from build123d import *

# Parameters (mm, degrees)
EXTRUDE1_DEPTH     = 50.8
SKETCH2_R          = 3.5687
CUT_EXTRUDE1_DEPTH = 7.3500001
SKETCH3_R          = 4.1656
CUT_EXTRUDE2_DEPTH = 128.0000001


with BuildPart() as part:
    # Sketch1 → Extrude1 (new body)
    with BuildSketch(Plane.XY):
        with BuildLine():
            Line((24.787766027, 20.626332144), (6.630852488, 23.827885887))
            Line((6.630852488, 23.827885887), (-1.306647512, 25.227481296))
            Line((-1.306647512, 25.227481296), (-11.14056344, 26.961466))
            add(Edge.make_bspline(
                [(-16.387897512, 33.214995232), (-16.387897512, 27.886712574), (-11.14056344, 26.961466)],
                knots=[1.570796327, 1.570796327, 1.570796327, 2.967059728, 2.967059728, 2.967059728], degree=2, weights=[1, 0.766044443, 1]))
            Line((-16.387897512, 33.214995232), (-16.387897512, 79.980278282))
            Line((-16.387897512, 79.980278282), (-16.387897512, 87.117678282))
            Line((-16.387897512, 87.117678282), (-16.387897512, 118.080278282))
            Line((-16.387897512, 118.080278282), (-16.387897512, 125.217678282))
            Line((-16.387897512, 125.217678282), (-16.387897512, 134.348978282))
            add(Edge.make_bspline(
                [(-16.387897512, 134.348978282), (-16.387897512, 140.698978282), (-22.737897512, 140.698978282)],
                knots=[3.141592654, 3.141592654, 3.141592654, 4.71238898, 4.71238898, 4.71238898], degree=2, weights=[1, 0.707106781, 1]))
            Line((-22.737897512, 140.698978282), (-22.737897512, 125.217678282))
            Line((-22.737897512, 125.217678282), (-22.737897512, 118.080278282))
            Line((-22.737897512, 118.080278282), (-22.737897512, 87.117678282))
            Line((-22.737897512, 87.117678282), (-22.737897512, 79.980278282))
            Line((-22.737897512, 79.980278282), (-22.737897512, 13.698978282))
            Line((-22.737897512, 13.698978282), (-1.306647512, 13.698978282))
            Line((-1.306647512, 13.698978282), (6.630852488, 13.698978282))
            Line((6.630852488, 13.698978282), (28.062102488, 13.698978282))
            Line((28.062102488, 13.698978282), (28.062102488, 16.724129903))
            add(Edge.make_bspline(
                [(28.062102488, 16.724129903), (28.062102488, 20.048978282), (24.787766027, 20.626332144)],
                knots=[0, 0, 0, 1.396263402, 1.396263402, 1.396263402], degree=2, weights=[1, 0.766044443, 1]))
        make_face()
    extrude(amount=EXTRUDE1_DEPTH)

    # Sketch2 → Cut-Extrude1 (cut, through all)
    with BuildSketch(Plane(origin=(-16.387897512, 0, 0), x_dir=(0, 0, -1), z_dir=(1, 0, 0))):
        with Locations((-38.1, 121.648978282)):
            Circle(SKETCH2_R)
        with Locations((-38.1, 83.548978282)):
            Circle(SKETCH2_R)
        with Locations((-12.685238078, 83.548978282)):
            Circle(SKETCH2_R)
        with Locations((-12.685238078, 121.64899544)):
            Circle(SKETCH2_R)
    extrude(amount=-CUT_EXTRUDE1_DEPTH, mode=Mode.SUBTRACT)

    # Sketch3 → Cut-Extrude2 (cut, through all)
    with BuildSketch(Plane.XZ.offset(-13.698978282)):
        with Locations((2.662102488, 12.7)):
            Circle(SKETCH3_R)
        with Locations((2.662102488, 38.1)):
            Circle(SKETCH3_R)
    extrude(amount=-CUT_EXTRUDE2_DEPTH, mode=Mode.SUBTRACT)


solid = part.part
The listing builds one solid part. Answer for the finished solid, in the listing's coordinates (mm). A direction names the side the tool comes from. Coordinates: 2 decimals unless noted, no trailing zeros. Loops run counter-clockwise (first coordinate to the right, second up) from the corner with the lowest first, then second, coordinate; pieces in that order, holes last. Notation, with made-up numbers: (45, 61) -> (90, 61) arc R33 cw to (90, 97) -> close; hole circle Ø6 at (8, 47.5). An arc over 180 degrees is marked (long way). Write item = value, one per line. Start each with the question number.
1) Straight lines are drawn through the part: line 1 (Y direction, x = -19.5, z = 38.1); line 2 (X direction, y = 47, z = 38); line 3 (Y direction, x = -19, z = 38). For each, find the intervals that lie inside material, in ascending order. Write a range as from..to.
2) A tool of negligible diameter and unlimited length cuts with its end or side. For faces 5 (the face through (-16.388, 83, 25)), 6 (the face through (-22.738, 78, 25)), from which of +Z, -Z, +X, -X, +Y, -Y can it reach the whole face along a straight path? Write none if from no direction.
3) A cutting plane is placed at A-A (y = 22.5). Give the vertices of the cut face in (x, z), then the cut area to 3 significant figures.
4) A cutting plane is placed at D-D (x = 11). Give the vertices of the cut face in (y, z), then the cut area to 3 significant figures.
5) A cutting plane is placed at B-B (y = 70). Give the vertices of the cut face in (x, z).
6) Given pin 1 Ø15 at (y, z) = (73, 34.5) entering from +X; pin 2 Ø5.5 at (y, z) = (83.55, 38.1) entering from +X; pin 3 Ø8 at (x, z) = (9, 20.5) entering from +Y; pin 4 Ø11 at (x, z) = (2.66, 12.7) entering from +Y, each flat-ended and moving along its own axis, determine where each tip first touches the part or whether it passes through.
7) The mould has two halves that part along Y. Classify faces 1 (the face through (2, 13.699, 25)), 2 (the face through (-18, 54, 50.8)), 3 (the face through (-19.518, 87.087, 38.565)), 4 (the face through (-19.518, 125.187, 38.565)): released by +Y, released by -Y, zero draft, split by the parting line, or undercut.
8) A cutting plane is placed at C-C (z = 38.1). Count the separate pieces of the cut face and the enclosed holes in it, then the cut area to 3 significant figures.
Responses:
q1.line_1 = 13.7..79.98, 87.12..118.08, 125.22..139.81
q1.line_2 = -22.74..-16.39
q1.line_3 = 13.7..79.98, 87.12..118.08, 125.22..139.48
q2.face_5 = +Z, -Z, +X, +Y
q2.face_6 = +Z, -Z, -X, +Y, -Y
q3.outline = (-22.74, 0) -> (14.16, 0) -> (14.16, 50.8) -> (-22.74, 50.8) -> close; hole circle Ø8.33 at (2.66, 12.7); hole circle Ø8.33 at (2.66, 38.1)
q3.area = 1,770 mm²
q4.outline = (13.7, 0) -> (23.06, 0) -> (23.06, 50.8) -> (13.7, 50.8) -> close
q4.area = 475 mm²
q5.outline = (-22.74, 0) -> (-16.39, 0) -> (-16.39, 50.8) -> (-22.74, 50.8) -> close
q6.pin_1 = -16.39
q6.pin_2 = through
q6.pin_3 = 24.12
q6.pin_4 = 25.5
q7.face_1 = released by -Y
q7.face_2 = zero draft
q7.face_3 = undercut
q7.face_4 = undercut
q8.separate_pieces = 4
q8.enclosed_holes = 0
q8.area = 1,080 mm²
